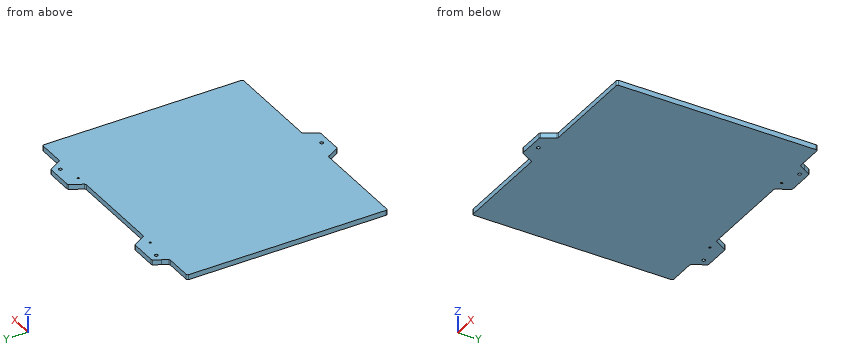
Autodesk Inventor part; units mm, degrees
ref_plane "YZ Plane" through (0, 0, 0) normal (1, 0, 0) x (0, 1, 0)
ref_plane "XZ Plane" through (0, 0, 0) normal (0, 1, 0) x (-1, 0, 0)
ref_plane "XY Plane" through (0, 0, 0) normal (0, 0, 1) x (1, 0, 0)
sketch "Sketch1" plane through (0, 0, 0) normal (0, 0, 1) x (1, 0, 0)
  line L0 (151, -126) -> (-151, -126)
  line L1 (-151, -126) -> (-151, 126)
  line L2 (-151, 126) -> (151, 126)
  line L3 (151, 126) -> (151, -126)
  line L4 (151, -126) -> (-151, 126) construction
  line L5 (-151, -126) -> (151, 126) construction
  point P0 (0, 0)
  dimension "d0" = 302
  dimension "d1" = 252
extrude "Extrusion1" add sketch "Sketch1" along normal blind 6.35
sketch "Sketch2" plane through (0, 0, 6.35) normal (0, 0, 1) x (1, 0, 0)
  line L0 (-110.3923, 134) -> (-105.1962, 143)
  line L1 (-105.1962, 143) -> (-94.8038, 143)
  line L2 (-94.8038, 143) -> (-89.6077, 134)
  line L3 (-89.6077, 134) -> (-94.8038, 125)
  line L4 (-94.8038, 125) -> (-105.1962, 125)
  line L5 (-105.1962, 125) -> (-110.3923, 134)
  line L6 (94.8038, 143) -> (105.1962, 143)
  line L7 (105.1962, 143) -> (110.3923, 134)
  line L8 (110.3923, 134) -> (105.1962, 125)
  line L9 (105.1962, 125) -> (94.8038, 125)
  line L10 (94.8038, 125) -> (89.6077, 134)
  line L11 (89.6077, 134) -> (94.8038, 143)
  line L12 (-100, 134) -> (100, 134) construction
  line L13 (151, 126) -> (-151, 126)
  line L14 (-105.1962, 143) -> (-115.0111, 126)
  line L15 (105.1962, 143) -> (115.0111, 126)
  line L16 (94.8038, 143) -> (-94.8038, 143)
  line L17 (-151, -126) -> (151, -126)
  line L18 (-27.315, -126) -> (-17.5, -143)
  line L19 (-17.5, -143) -> (17.5, -143)
  line L20 (17.5, -143) -> (27.315, -126)
  line L21 (-70.1962, 143) -> (-60.3812, 126)
  line L22 (60.3812, 126) -> (70.1962, 143)
  point P0 (0, 0)
  point P1 (0, 134)
  point P2 (0, -143)
  point P3 (0, -134)
  dimension "d4" = 18
  dimension "d5" = 200
  dimension "d6" = 8
  dimension "d7" = 17
  dimension "d8" = 17
  dimension "d9" = 35
  dimension "d10" = 8
  dimension "d32" = 35
  dimension "d33" = 35
extrude "Extrusion2" add sketch "Sketch2" against normal up to surface (6.35 mm away) contours L0 L1 L2 L3 L13 L5 | L5 L13 L14 | L16 L21 L13 L3 L2 | L16 L11 L10 L13 L22 | L6 L7 L8 L13 L10 L11 | L8 L15 L13 | L17 L20 L19 L18
hole "Hole1" at (0, -134, 6.35) at (-100, 134, 6.35) at (100, 134, 6.35) direction (0, 0, -1) diameter 4.134 end through all
fillet "Fillet1" radius 2 16 edges at (17.5, -143, 3.175) (27.315, -126, 3.175) (151, -126, 3.175) (-151, 126, 3.175) (115.0111, 126, 3.175) (105.1962, 143, 3.175) (151, 126, 3.175) (-27.315, -126, 3.175) (-17.5, -143, 3.175) (-151, -126, 3.175) (-115.0111, 126, 3.175) (-105.1962, 143, 3.175) (-70.1962, 143, 3.175) (-60.3812, 126, 3.175) (60.3812, 126, 3.175) (70.1962, 143, 3.175)
sketch "Sketch3" plane through (0, 0, 6.35) normal (0, 0, 1) x (1, 0, 0)
  line L0 (150, -125) -> (-150, -125) construction
  line L1 (-150, -125) -> (-150, 125) construction
  line L2 (-150, 125) -> (150, 125) construction
  line L3 (150, 125) -> (150, -125) construction
  line L4 (150, -125) -> (-150, 125) construction
  line L5 (-150, -125) -> (150, 125) construction
  circle A0 centre (-75, 126.6) radius 1.6 construction
  line L6 (-75, 126.6) -> (75, 126.6) construction
  circle A1 centre (75, 126.6) radius 1.6 construction
  point P0 (0, 0)
  point P1 (0, 126.6)
  dimension "d21" = 300
  dimension "d22" = 250
  dimension "d23" = 3.2
  dimension "d24" = 150
hole "Hole2" at (-75, 126.6, 6.35) at (75, 126.6, 6.35) direction (0, 0, -1) diameter 2.459 end through all
equation "\"d7\" = d8"
equation "\"d32\" = d9"
equation "\"d33\" = d32"
properties part number "Print Bed" material "Aluminum 6061"
Model file for the job. Use its own axes, mm. Round coordinates to 2 decimals unless told otherwise and drop trailing zeros. Loops run counter-clockwise (first coordinate to the right, second up) from the corner with the lowest first, then second, coordinate; pieces in that order, holes last. Notation, with made-up numbers: (42.25, 32) -> (69.25, 32) arc R12 cw to (69.25, 54) -> close; hole circle Ø2 at (76.5, 72). An arc over 180 degrees is marked (long way). Answer as CSV lines item,"result". Start each with the question number.
1) Probe line 1 along Y through (x, z) = (0, 3.25); line 2 along X through (y, z) = (134, 4.5); line 3 along Y through (x, z) = (-100, 3.5). List the from-to ranges inside material, lowest first.
2) Pin check, flat tip, straight feed: P1, Ø3, axis at x = 16, z = 2, coming from the +Y side. Stop position of the tip, or through.
3) Slice it at B-B (z = 3.5). State how many separate pieces and enclosed holes the cut face has, plus the area to 3 significant figures.
4) Slice it at C-C (x = -41.5). List the corners of the cut face in (y, z).
5) Slice it at A-A (x = -93). List the corners of the cut face in (y, z).
Filled in:
1,line 1,"y = -143 to -136.07, -131.93 to 126"
1,line 2,"x = -110.39 to -102.07, -97.93 to -65, 65 to 97.93, 102.07 to 110.39"
1,line 3,"y = -126 to 131.93, 136.07 to 143"
2,P1,"stops at y = 126"
3,separate pieces,"1"
3,enclosed holes,"5"
3,area,"78,300 mm2"
4,outline,"(-126, 0) -> (126, 0) -> (126, 6.35) -> (-126, 6.35) -> close"
5,outline,"(-126, 0) -> (143, 0) -> (143, 6.35) -> (-126, 6.35) -> close"
